from build123d import *

# Parameters (mm, degrees)
EXTRUDE_1_DEPTH     = 49.8
CHAMFER_1_SIZE      = 5
SKETCH_3_W          = 0.807071686
SKETCH_3_H          = 22.587877847
CUT_EXTRUDE_1_DEPTH = 49.8


with BuildPart() as part:
    # 草图1 → 凸台-拉伸1 (new body)
    with BuildSketch(Plane(origin=(0, 0, 0), x_dir=(0, 0, -1), z_dir=(1, 0, 0))):
        with BuildLine():
            Line((-3.30116432, 4.869061466), (-14.31163185, 4.869061466))
            Line((-14.31163185, 4.869061466), (-14.31163185, -2.159184752))
            ThreePointArc((-14.31163185, -2.159184752), (-13.694314645, -3.083064362), (-12.604524306, -2.866290096))
            Line((-12.604524306, -2.866290096), (-10.135977537, -0.42662706))
            ThreePointArc((-10.135977537, -0.42662706), (-10.00408666, -0.265887616), (-9.841806105, -0.13589764))
            ThreePointArc((-9.841806105, -0.13589764), (-8.821917683, -0.099462208), (-8.30116432, -0.977138612))
            Line((-8.30116432, -0.977138612), (-8.30116432, -3.015902523))
            Line((-8.30116432, -3.015902523), (-8.30116432, -8.640917782))
            Line((-8.30116432, -8.640917782), (-3.30116432, -8.640917782))
            Line((-3.30116432, -8.640917782), (-3.30116432, 4.869061466))
        make_face()
        with BuildLine():
            ThreePointArc((-8.30116432, 10.715261544), (-8.821917683, 9.83758514), (-9.841806105, 9.874020573))
            ThreePointArc((-9.841806105, 9.874020573), (-10.00408666, 10.004010548), (-10.135977537, 10.164749992))
            Line((-10.135977537, 10.164749992), (-12.604524306, 12.604413029))
            ThreePointArc((-12.604524306, 12.604413029), (-13.694314645, 12.821187294), (-14.31163185, 11.897307685))
            Line((-14.31163185, 11.897307685), (-14.31163185, 4.869061466))
            Line((-14.31163185, 4.869061466), (-3.30116432, 4.869061466))
            Line((-3.30116432, 4.869061466), (-3.30116432, 13.139889713))
            Line((-3.30116432, 13.139889713), (-5.608236006, 15.446957584))
            Line((-5.608236006, 15.446957584), (-8.30116432, 12.754025455))
            Line((-8.30116432, 12.754025455), (-8.30116432, 10.715261544))
        make_face()
    extrude(amount=EXTRUDE_1_DEPTH)

    # 倒角1
    chamfer_1_edges = [part.edges().sort_by_distance(p)[0] for p in [
        (0, -8.640917782, 5.80116432),
        (49.8, -8.640917782, 5.80116432),
    ]]
    chamfer(chamfer_1_edges, length=CHAMFER_1_SIZE)

    # 草图3 → 切除-拉伸1 (cut)
    with BuildSketch(Plane(origin=(49.8, 0, 0), x_dir=(0, 0, -1), z_dir=(1, 0, 0))):
        with Locations((-3.704700163, 2.653021142)):
            Rectangle(SKETCH_3_W, SKETCH_3_H)
    extrude(amount=-CUT_EXTRUDE_1_DEPTH, mode=Mode.SUBTRACT)


solid = part.part
Verification items for the finished model (mm, model axes). A direction names the side the tool comes from. Round coordinates to 2 decimals unless told otherwise and drop trailing zeros. Order: outer loops, then holes, each group sorted by start corner. A loop starts at its lowest first (then second) coordinate and runs counter-clockwise, first axis right, second up. Notation, with made-up numbers: (64.25, -18) -> (89.25, -18) arc R17 ccw to (89.25, 11) -> close; hole circle Ø8 at (73, 41). An arc over 180 degrees is marked (long way). Put each result on its own line as item: value.
1) Material ranges on line 1 (Z direction, x = 34, y = -6.75); line 2 (Z direction, x = 16.5, y = -1.25); line 3 (Y direction, x = 41, z = 6.75), recorded low to high.
Final values:
line 1: z = 4.11 to 8.3
line 2: z = 4.11 to 8.3, 10.97 to 14.31
line 3: y = -8.64 to 14.31
2) Section check A-A (x = 35). Record the cut outline in (y, z).
Final values:
outline: (-8.64, 4.11) -> (13.95, 4.11) -> (15.45, 5.61) -> (12.75, 8.3) -> (10.72, 8.3) arc R1 cw to (10.16, 10.14) -> (12.6, 12.6) arc R1 ccw to (11.9, 14.31) -> (-2.16, 14.31) arc R1 ccw to (-2.87, 12.6) -> (-0.43, 10.14) arc R1 cw to (-0.98, 8.3) -> (-8.64, 8.3) -> close
3) Mould release check, pull along Z, two halves, no side actions. Record for faces 1 (the flat face through (25, 5, 14.312)), 2 (the flat face through (25, 2, 4.108)), 3 (the flat face through (24.551, 11.368, 11.353)), 4 (the flat face through (49.8, 6, 9)): +Z half, -Z half, draft (parallel to the pull), parting line (faces both ways), or undercut.
Final values:
face 1: +Z half
face 2: -Z half
face 3: undercut
face 4: draft
4) Section check D-D (z = 12). Record the cut outline in (x, y), then the cut area to 3 significant figures.
Final values:
outline: (0, -2.27) -> (49.8, -2.27) -> (49.8, 12.01) -> (0, 12.01) -> close
area: 711 mm^2
5) Section check C-C (y = -5.5). Record the cut outline in (x, z), then the cut area to 3 significant figures.
Final values:
outline: (1.86, 4.11) -> (47.94, 4.11) -> (47.94, 8.3) -> (1.86, 8.3) -> close
area: 193 mm^2
6) Section check B-B (z = 7). Record the cut outline in (x, y), then the cut area to 3 significant figures.
Final values:
outline: (0, -3.64) -> (5, -8.64) -> (44.8, -8.64) -> (49.8, -3.64) -> (49.8, 14.06) -> (0, 14.06) -> close
area: 1,110 mm^2
7) Depth check by flat-ended pin: pin 1 (2 mm diameter, centred on x = 17.5, z = 9.5, fed in from -Y); pin 2 (4 mm diameter, centred on x = 27.5, y = -5.5, fed in from +Z); pin 3 (1.5 mm diameter, centred on x = 27.5, z = 13, fed in from +Y). Enter the tip coordinate at first touch or a pass-through.
Final values:
pin 1: stops at y = -0.79
pin 2: stops at z = 8.3
pin 3: stops at y = 12.9
8) Set-up check for faces 5 (the flat face through (24.551, -1.664, 11.388)), 6 (the flat face through (25, 12, 8.301)), 7 (the flat face through (25, -8.641, 6)): record each of +Z, -Z, +X, -X, +Y, -Y from which the full face is reachable in a straight line by a thin tool's end or side.
Final values:
face 5: +X, -X, -Y
face 6: +X, -X, +Y
face 7: +Z, -Z, +X, -X, -Y
